Check sheet for the drawn part. Datum: minimum x, y, z corner. Units: mm. A direction names the side the tool comes from. Coordinates: 2 decimals unless noted, no trailing zeros. Loops run counter-clockwise (first coordinate to the right, second up) from the corner with the lowest first, then second, coordinate; pieces in that order, holes last. Notation, with made-up numbers: (31.25, 89) -> (81.25, 89) arc R28 cw to (81.25, 109) -> close; hole circle Ø2 at (32, 61.25). An arc over 180 degrees is marked (long way). Use CSV: the item, a comma, the result in double quotes. Start each with the question number.
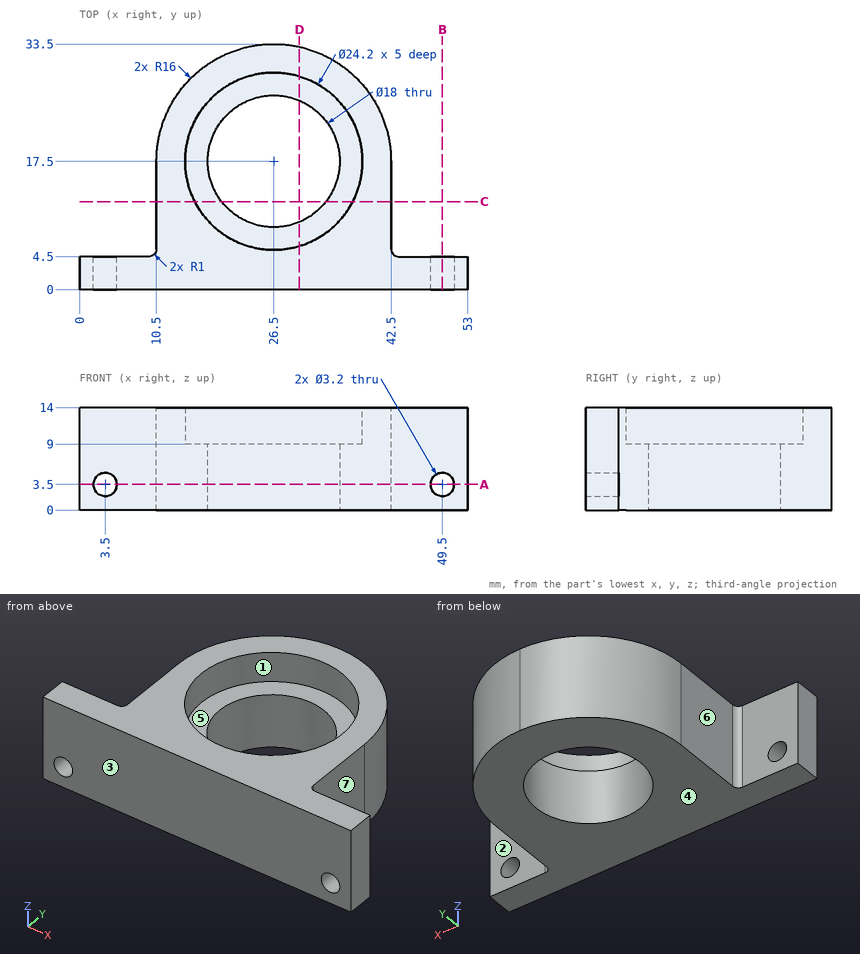
1. Set-up check for the marked faces 5, 6 and 7: record each of +Z, -Z, +X, -X, +Y, -Y from which the full face is reachable in a straight line by a thin tool's end or side.
2. Scan lines: line 1 (X direction, y = 3.3, z = 3.5); line 2 (Z direction, x = 3.5, y = 1.65); line 3 (Y direction, x = 26.5, z = 3). Record each from-to range of solid material in increasing order.
3. Cross-section at D-D, the plane x = 30. Record the boundary of the cut face in (y, z), plus the area to 4 significant figures.
4. Depth check by flat-ended pin: pin 1 (4 mm diameter, centred on x = 15.5, z = 4.5, fed in from -Y); pin 2 (6 mm diameter, centred on y = 18, z = 6, fed in from -X); pin 3 (4 mm diameter, centred on y = 14, z = 7, fed in from +X); pin 4 (3 mm diameter, centred on x = 5.5, z = 5.5, fed in from +Y). Enter the tip coordinate at first touch or a pass-through.
5. Release check for a two-part mould opening along Y. For the marked faces 1, 2, 3 and 4 record: released by +Y, released by -Y, zero draft, split by the parting line, or undercut.
6. Cross-section at B-B, the plane x = 49.5. Record the boundary of the cut face in (y, z).
7. Cross-section at A-A, the plane z = 3.5. State how many separate pieces and enclosed holes the cut face has, plus the area to 3 significant figures.
8. Cross-section at C-C, the plane y = 12. Record the boundary of the cut face in (x, z), plus the area to 3 significant figures.
Solution:
1,face 5,"+Z"
1,face 6,"+Z, -Z, -X, +Y"
1,face 7,"+Z, -Z, +X, +Y"
2,line 1,"x = 0 to 1.9, 5.1 to 47.9, 51.1 to 53"
2,line 2,"z = 0 to 1.9, 5.1 to 14"
2,line 3,"y = 0 to 8.5, 26.5 to 33.5"
3,outline,"(0, 0) -> (9.21, 0) -> (9.21, 9) -> (5.92, 9) -> (5.92, 14) -> (0, 14) -> close; (25.79, 0) -> (33.11, 0) -> (33.11, 14) -> (29.08, 14) -> (29.08, 9) -> (25.79, 9) -> close"
3,area,"198.5 mm2"
4,pin 1,"stops at y = 0"
4,pin 2,"stops at x = 10.5"
4,pin 3,"stops at x = 42.5"
4,pin 4,"stops at y = 4.5"
5,face 1,"undercut"
5,face 2,"released by +Y"
5,face 3,"released by -Y"
5,face 4,"zero draft"
6,outline,"(0, 0) -> (4.5, 0) -> (4.5, 1.9) -> (0, 1.9) -> close; (0, 5.1) -> (4.5, 5.1) -> (4.5, 14) -> (0, 14) -> close"
7,separate pieces,"3"
7,enclosed holes,"1"
7,area,"774 mm2"
8,outline,"(10.5, 0) -> (19.38, 0) -> (19.38, 9) -> (15.72, 9) -> (15.72, 14) -> (10.5, 14) -> close; (33.62, 0) -> (42.5, 0) -> (42.5, 14) -> (37.28, 14) -> (37.28, 9) -> (33.62, 9) -> close"
8,area,"212 mm2"
